Here's the drawing with two shaded views (mm, measured from the low corner). I have some questions. A direction names the side the tool comes from. Round coordinates to 2 decimals unless told otherwise and drop trailing zeros. Write each loop counter-clockwise with the first axis right and the second up, starting at its lowest first coordinate (ties: lowest second). Pieces come first, ordered by that corner, then holes. Notation, with made-up numbers: M 16,12 L 75,12 A21 cw 75,25 Z; hole C 58.5,-28.5 d10. An arc over 180 degrees is marked long. Write item = value, one per line. Start each with the question number.
(1) Will these pins go through, and if not, where does the flat tip stop? pin 1 Ø1.5 at (x, z) = (10, 3.5) entering from -Y; pin 2 Ø6 at (x, y) = (7.5, 8) entering from -Z; pin 3 Ø1 at (x, z) = (6.5, 3.5) entering from +Y; pin 4 Ø1 at (x, z) = (8, 7) entering from -Y.
(2) I need wall thicknesses on line 1 along X through (y, z) = (1.6, 3.5); line 2 along X through (y, z) = (2.25, 6.25); line 3 along Y through (x, z) = (7, 7.7). Which ranges of each line are inside material? Lowest first, please.
(3) I want a section at B-B (x = 7). List the corners of the cut face in (y, z) for me, and give its area (3 significant figures).
(4) If we mould it in two halves opening along Z, with no side actions, what happens to the marked faces 1, 2, 3 and 4? For each: released by +Z, released by -Z, zero draft, split by the parting line, or undercut.
(5) I want a section at A-A (z = 3.5). List the corners of the cut face in (x, y) for me.
(6) I want a section at D-D (y = 2.25). List the corners of the cut face in (x, z) for me.
(7) I want a section at C-C (y = 8). List the corners of the cut face in (x, z) for me.
(8) On a 3-axis mill with a long thin cutter (end or side, diameter ignored), from which of +Z, -Z, +X, -X, +Y, -Y can I reach the whole of each face in a straight line? I mean the marked faces 5 and 6. Say none if no direction works.
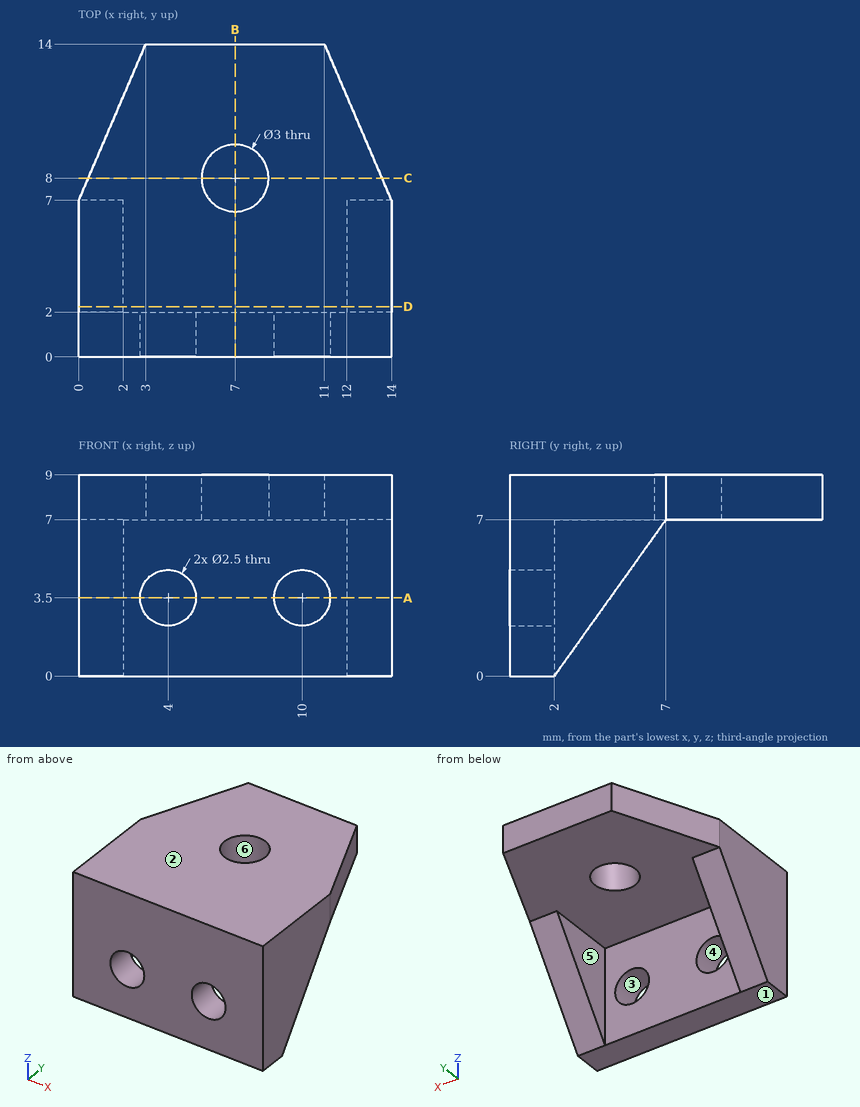
Returned:
q1.pin_1 = through
q1.pin_2 = 7
q1.pin_3 = 2
q1.pin_4 = 0
q2.line_1 = 0 to 2.75, 5.25 to 8.75, 11.25 to 14
q2.line_2 = 0 to 2, 12 to 14
q2.line_3 = 0 to 6.5, 9.5 to 14
q3.outline = M 0,0 L 2,0 L 2,7 L 6.5,7 L 6.5,9 L 0,9 Z; M 9.5,7 L 14,7 L 14,9 L 9.5,9 Z
q3.area = 36.0 mm²
q4.face_1 = released by -Z
q4.face_2 = released by +Z
q4.face_3 = undercut
q4.face_4 = undercut
q5.outline = M 0,0 L 2.75,0 L 2.75,2 L 2,2 L 2,4.5 L 0,4.5 Z; M 5.25,0 L 8.75,0 L 8.75,2 L 5.25,2 Z; M 11.25,0 L 14,0 L 14,4.5 L 12,4.5 L 12,2 L 11.25,2 Z
q6.outline = M 0,0.35 L 2,0.35 L 2,7 L 12,7 L 12,0.35 L 14,0.35 L 14,9 L 0,9 Z
q7.outline = M 0.43,7 L 5.5,7 L 5.5,9 L 0.43,9 Z; M 8.5,7 L 13.57,7 L 13.57,9 L 8.5,9 Z
q8.face_5 = -Z, +Y
q8.face_6 = +Z, -Z
